```python
from build123d import *

# Parameters (mm, degrees)
SKETCH1_W           = 22.5
SKETCH1_H           = 12.6
BOSS_EXTRUDE1_DEPTH = 16
SHELL2_T            = 1
SKETCH2_R           = 1
BOSS_EXTRUDE2_DEPTH = 1.5
SKETCH5_W           = 17
SKETCH5_H           = 1.5
BOSS_EXTRUDE3_DEPTH = 10
SKETCH6_W           = 17
SKETCH6_H           = 11.6
BOSS_EXTRUDE4_DEPTH = 2


with BuildPart() as part:
    # Sketch1 → Boss-Extrude1 (new body)
    with BuildSketch(Plane.XY):
        Rectangle(SKETCH1_W, SKETCH1_H)
    extrude(amount=BOSS_EXTRUDE1_DEPTH)

    # Shell2
    shell2_openings = [part.faces().sort_by_distance(p)[0] for p in [
        (0, 0, 0),
    ]]
    offset(amount=SHELL2_T, openings=shell2_openings, kind=Kind.INTERSECTION)

    # Sketch2 → Boss-Extrude2 (add)
    with BuildSketch(Plane(origin=(0, 0, 0), x_dir=(-1, 0, 0), z_dir=(0, 0, -1))):
        with BuildLine():
            Line((-13.45, -4.2), (-13.25, -4.2))
            ThreePointArc((-13.25, -4.2), (-12.542893219, -4.492893219), (-12.25, -5.2))
            Line((-12.25, -5.2), (-12.25, 4.8))
            ThreePointArc((-12.25, 4.8), (-12.542893219, 4.092893219), (-13.25, 3.8))
            Line((-13.25, 3.8), (-13.45, 3.8))
            ThreePointArc((-13.45, 3.8), (-14.864213562, 3.214213562), (-15.45, 1.8))
            Line((-15.45, 1.8), (-15.45, -2.2))
            ThreePointArc((-15.45, -2.2), (-14.864213562, -3.614213562), (-13.45, -4.2))
        make_face()
        with Locations((-13.85, 0)):
            Circle(SKETCH2_R, mode=Mode.SUBTRACT)
    boss_extrude2 = extrude(amount=-BOSS_EXTRUDE2_DEPTH)

    # Mirror1: Boss-Extrude2 across plane
    add(boss_extrude2.mirror(Plane(origin=(0, 0, 0), x_dir=(0, 0, 1), z_dir=(1, 0, 0))))

    # Sketch5 → Boss-Extrude3 (add)
    with BuildSketch(Plane.ZY.offset(12.25)):
        with Locations((8.5, 6.55)):
            Rectangle(SKETCH5_W, SKETCH5_H)
        with Locations((8.5, -6.55)):
            Rectangle(SKETCH5_W, SKETCH5_H)
    extrude(amount=BOSS_EXTRUDE3_DEPTH)

    # Sketch6 → Boss-Extrude4 (add)
    with BuildSketch(Plane.ZY.offset(22.25)):
        with Locations((8.5, 0)):
            Rectangle(SKETCH6_W, SKETCH6_H)
    extrude(amount=-BOSS_EXTRUDE4_DEPTH)


solid = part.part
```
Geometry check sheet. Reference: the model listing, model coordinates, mm. A direction names the side the tool comes from. Give positions to 0.01 mm unless a question says otherwise; leave off trailing zeros. Order: outer loops, then holes, each group sorted by start corner. A loop starts at its lowest first (then second) coordinate and runs counter-clockwise, first axis right, second up.
1. Thickness scan on L1, parallel to X at y = 3.5, z = 7.5; L2, parallel to Y at x = -16, z = 1.25; L3, parallel to X at y = 6, z = 1.5. Record the ranges inside material, lowest first.
2. Release check for a two-part mould opening along Y. For faces 1 (the face through (14.88, -3.6, 0.74)), 2 (the face through (14.85, 0.04, 0.74)), 3 (the face through (12.25, 0, 8)) record: pulls with the +Y half, pulls with the -Y half, needs draft (parallel to the pull), parting line crosses it, or undercut.
3. Section check D-D, the plane x = -13.85. Enter the section's corners in (y, z).
4. Access from +Z, -Z, +X, -X, +Y, -Y to the whole of each face (thin tool, end or side, straight path). Record for faces 4 (the face through (-5, -7.3, 8)), 5 (the face through (-15.45, 0, 1)), 6 (the face through (-12.25, 0, 8)), 7 (the face through (-12, 0, 0)), 8 (the face through (0, -6.3, 8)).
5. Section check A-A, the plane x = -19. Enter the section's corners in (y, z), and give its area (3 significant figures).
6. Section check C-C, the plane z = 10. Enter the section's corners in (x, y), and give its area (3 significant figures).
7. Section check B-B, the plane y = 0. Enter the section's corners in (x, z), and give its area (3 significant figures).
8. Gauge pin test, flat ends, axial feed: pin 1 Ø1 at (y, z) = (-5, 12.5) entering from +X; pin 2 Ø1 at (x, y) = (13, 2) entering from +Z. Record the tip position at first contact, or that the pin passes through.
Values follow:
1. L1: x = -22.25 to -20.25, -12.25 to -11.25, 11.25 to 12.25
1. L2: y = -7.3 to -5.8, 5.8 to 7.3
1. L3: x = -22.25 to -11.25, 11.25 to 12.25
2. face 1: pulls with the -Y half
2. face 2: undercut
2. face 3: needs draft
3. outline: (-7.3, 0) - (-5.8, 0) - (-5.8, 17) - (-7.3, 17) - close; (-4.16, 0) - (-1, 0) - (-1, 1.5) - (-4.16, 1.5) - close; (1, 0) - (3.76, 0) - (3.76, 1.5) - (1, 1.5) - close; (5.8, 0) - (7.3, 0) - (7.3, 17) - (5.8, 17) - close
4. face 4: +Z, -Z, +X, -X, -Y
4. face 5: +Z, -Z
4. face 6: +Z
4. face 7: -Z, +X, -X, +Y, -Y
4. face 8: -Z
5. outline: (-7.3, 0) - (-5.8, 0) - (-5.8, 17) - (-7.3, 17) - close; (5.8, 0) - (7.3, 0) - (7.3, 17) - (5.8, 17) - close
5. area: 51.0 mm2
6. outline: (-22.25, -7.3) - (12.25, -7.3) - (12.25, 7.3) - (-22.25, 7.3) - close; hole (-20.25, -5.8) - (-12.25, -5.8) - (-12.25, 5.8) - (-20.25, 5.8) - close; hole (-11.25, -6.3) - (11.25, -6.3) - (11.25, 6.3) - (-11.25, 6.3) - close
6. area: 127 mm2
7. outline: (-22.25, 0) - (-20.25, 0) - (-20.25, 17) - (-22.25, 17) - close; (-15.45, 0) - (-14.85, 0) - (-14.85, 1.5) - (-15.45, 1.5) - close; (-12.85, 0) - (-11.25, 0) - (-11.25, 16) - (11.25, 16) - (11.25, 0) - (12.85, 0) - (12.85, 1.5) - (12.25, 1.5) - (12.25, 17) - (-12.25, 17) - (-12.25, 1.5) - (-12.85, 1.5) - close; (14.85, 0) - (15.45, 0) - (15.45, 1.5) - (14.85, 1.5) - close
7. area: 94.1 mm2
8. pin 1: stops at x = 12.25
8. pin 2: stops at z = 1.5
